from build123d import *

# Parameters (mm, degrees)
SKETCH2_W           = 42.3
SKETCH2_H           = 42.3
BOSS_EXTRUDE1_DEPTH = 32.5
CHAMFER1_SIZE       = 5.5
SKETCH3_R           = 11
SKETCH3_R_2         = 3.430858596
BOSS_EXTRUDE2_DEPTH = 1.5
SKETCH4_R           = 16
SKETCH4_R_2         = 11
CUT_EXTRUDE1_DEPTH  = 0.3
SKETCH5_R           = 1.5
BOSS_EXTRUDE3_DEPTH = 25.4


with BuildPart() as part:
    # Sketch2 → Boss-Extrude1 (new body)
    with BuildSketch(Plane(origin=(0, 0, 0), x_dir=(1, 0, 0), z_dir=(0, 1, 0))):
        Rectangle(SKETCH2_W, SKETCH2_H)
    extrude(amount=BOSS_EXTRUDE1_DEPTH)

    # Chamfer1
    chamfer1_edges = [part.edges().sort_by_distance(p)[0] for p in [
        (21.15, 16.25, 21.15),
        (-21.15, 16.25, 21.15),
        (-21.15, 16.25, -21.15),
        (21.15, 16.25, -21.15),
    ]]
    chamfer(chamfer1_edges, length=CHAMFER1_SIZE)

    # Sketch3 → Boss-Extrude2 (add)
    with BuildSketch(Plane(origin=(0, 32.5, 0), x_dir=(1, 0, 0), z_dir=(0, 1, 0))):
        Circle(SKETCH3_R)
        Circle(SKETCH3_R_2, mode=Mode.SUBTRACT)
    extrude(amount=BOSS_EXTRUDE2_DEPTH)

    # Sketch4 → Cut-Extrude1 (cut)
    with BuildSketch(Plane(origin=(0, 32.5, 0), x_dir=(1, 0, 0), z_dir=(0, 1, 0))):
        Circle(SKETCH4_R)
        Circle(SKETCH4_R_2, mode=Mode.SUBTRACT)
    extrude(amount=-CUT_EXTRUDE1_DEPTH, mode=Mode.SUBTRACT)

    # Sketch5 → Boss-Extrude3 (add)
    with BuildSketch(Plane(origin=(0, 32.5, 0), x_dir=(1, 0, 0), z_dir=(0, 1, 0))):
        Circle(SKETCH5_R)
    extrude(amount=BOSS_EXTRUDE3_DEPTH)


solid = part.part
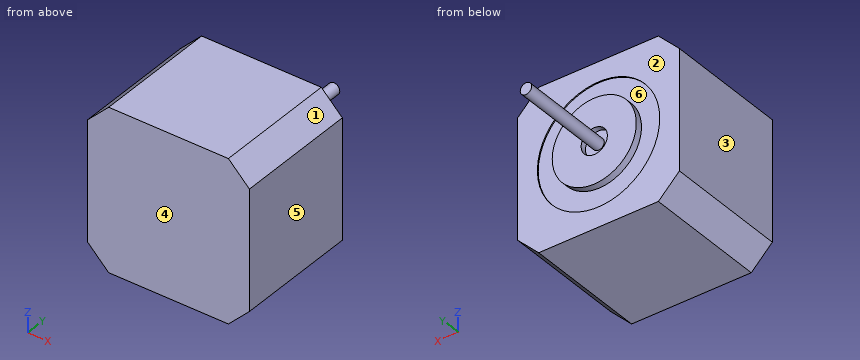
Geometry: final body of the model. Coordinates: model frame, mm. Face numbers are marked on the shaded views. A direction names the side the tool comes from. Round coordinates to 2 decimals unless told otherwise and drop trailing zeros. Order: outer loops, then holes, each group sorted by start corner. A loop starts at its lowest first (then second) coordinate and runs counter-clockwise, first axis right, second up. Notation, with made-up numbers: (-14, 88) - (41, 88) arc R20 cw to (41, 121) - close; hole circle Ø4 at (76.25, -12.75). An arc over 180 degrees is marked (long way). Write each question's results on one line, items separated by ' | '.
Item 1: Reachability of the marked faces 1 and 2 from +Z, -Z, +X, -X, +Y, -Y: full face, straight path, thin tool, end or side. Return the list, or none.
Completed:
face 1: +Z, +X, +Y, -Y | face 2: +Y
Item 2: First-contact query: pin 1 Ø2 at (x, y) = (-17, 19.5) entering from -Z; pin 2 Ø6 at (x, y) = (2, 40) entering from +Z; pin 3 Ø4 at (x, z) = (-14.5, 5.5) entering from +Y. Flat tips, straight axial feed; report the tip coordinate or a pass-through.
Completed:
pin 1: z = -20.8 | pin 2: z = 1.5 | pin 3: y = 32.5
Item 3: Section A-A, the plane x = 0. Return the cut outline in (y, z), and give its area (3 significant figures).
Completed:
outline: (0, -21.15) - (32.5, -21.15) - (32.5, -16) - (32.2, -16) - (32.2, -11) - (34, -11) - (34, -3.43) - (32.5, -3.43) - (32.5, -1.5) - (57.9, -1.5) - (57.9, 1.5) - (32.5, 1.5) - (32.5, 3.43) - (34, 3.43) - (34, 11) - (32.2, 11) - (32.2, 16) - (32.5, 16) - (32.5, 21.15) - (0, 21.15) - close | area: 1,470 mm^2
Item 4: Material intervals for line 1 along Z through (x, y) = (0, 32.4); line 2 along Z through (x, y) = (0, 33.15), sorted ascending. Write a range as [from, to].
Completed:
line 1: [-21.15, -16], [-11, 11], [16, 21.15] | line 2: [-11, -3.43], [-1.5, 1.5], [3.43, 11]
Item 5: Section D-D, the plane z = -12. Return the cut outline in (x, y), and give its area (3 significant figures).
Completed:
outline: (-21.15, 0) - (21.15, 0) - (21.15, 32.5) - (10.58, 32.5) - (10.58, 32.2) - (-10.58, 32.2) - (-10.58, 32.5) - (-21.15, 32.5) - close | area: 1,370 mm^2
Item 6: Mould query, pull axis X, two halves, no side actions, for the marked faces 3, 4, 5 and 6. Classes: pulls with the +X half, pulls with the -X half, needs draft (parallel to the pull), parting line crosses it, or undercut.
Completed:
face 3: pulls with the -X half | face 4: needs draft | face 5: pulls with the +X half | face 6: undercut
Item 7: Section C-C, the plane y = 21. Return the cut outline in (x, z).
Completed:
outline: (-21.15, -15.65) - (-15.65, -21.15) - (15.65, -21.15) - (21.15, -15.65) - (21.15, 15.65) - (15.65, 21.15) - (-15.65, 21.15) - (-21.15, 15.65) - close
Item 8: Section B-B, the plane z = 0. Return the cut outline in (x, y).
Completed:
outline: (-21.15, 0) - (21.15, 0) - (21.15, 32.5) - (16, 32.5) - (16, 32.2) - (11, 32.2) - (11, 34) - (3.43, 34) - (3.43, 32.5) - (1.5, 32.5) - (1.5, 57.9) - (-1.5, 57.9) - (-1.5, 32.5) - (-3.43, 32.5) - (-3.43, 34) - (-11, 34) - (-11, 32.2) - (-16, 32.2) - (-16, 32.5) - (-21.15, 32.5) - close
